```python
from build123d import *

# Parameters (mm, degrees)
BOSS_EXTRUDE2_DEPTH = 10
SKETCH2_W           = 6
SKETCH2_H           = 21.5
CUT_EXTRUDE1_DEPTH  = 2
SKETCH18_W          = 10
SKETCH18_H          = 4
CUT_EXTRUDE6_DEPTH  = 2.32
BOSS_EXTRUDE4_DEPTH = 35.965
SKETCH20_W          = 10
SKETCH20_H          = 4.318
BOSS_EXTRUDE5_DEPTH = 9
SKETCH21_W          = 2
SKETCH21_H          = 57.465
BOSS_EXTRUDE6_DEPTH = 0.889
BOSS_EXTRUDE7_DEPTH = 9.02
CUT_EXTRUDE7_DEPTH  = 1.016
SKETCH24_W          = 4.069
SKETCH24_H          = 2.54
CUT_EXTRUDE8_DEPTH  = 1
SKETCH30_R          = 0.75565
CUT_EXTRUDE14_DEPTH = 95.738007626
SKETCH34_R          = 1.5
CUT_EXTRUDE18_DEPTH = 10
SKETCH35_R          = 0.75
CUT_EXTRUDE19_DEPTH = 60.59814159
SKETCH36_W          = 6
SKETCH36_H          = 10
CUT_EXTRUDE20_DEPTH = 10
SKETCH37_W          = 9
SKETCH37_H          = 2
BOSS_EXTRUDE8_DEPTH = 3.65
SKETCH38_W          = 4.069
SKETCH38_H          = 10
BOSS_EXTRUDE9_DEPTH = 3
SKETCH39_R          = 0.75
CUT_EXTRUDE21_DEPTH = 3


with BuildPart() as part:
    # Sketch1 → Boss-Extrude2 (new body)
    with BuildSketch(Plane.XY):
        Polygon((-4, 0), (-0.82, 0), (-0.82, 21.5), (-6.32, 21.5), (-6.32, 17.5), (-4, 17.5), align=None)
    extrude(amount=BOSS_EXTRUDE2_DEPTH)

    # Sketch2 → Cut-Extrude1 (cut)
    with BuildSketch(Plane(origin=(-0.82, 0, 0), x_dir=(0, 0, -1), z_dir=(1, 0, 0))):
        with Locations((-5, 10.75)):
            Rectangle(SKETCH2_W, SKETCH2_H)
    extrude(amount=-CUT_EXTRUDE1_DEPTH, mode=Mode.SUBTRACT)

    # Sketch18 → Cut-Extrude6 (cut)
    with BuildSketch(Plane.ZY.offset(6.32)):
        with Locations((5, 19.5)):
            Rectangle(SKETCH18_W, SKETCH18_H)
    extrude(amount=-CUT_EXTRUDE6_DEPTH, mode=Mode.SUBTRACT)

    # Sketch19 → Boss-Extrude4 (add)
    with BuildSketch(Plane(origin=(0, 21.5, 0), x_dir=(1, 0, 0), z_dir=(0, 1, 0))):
        Polygon((-0.82, -10), (-4, -10), (-4, 0), (-0.82, 0), (-0.82, -2), (-2.82, -2), (-2.82, -8), (-0.82, -8), align=None)
    extrude(amount=BOSS_EXTRUDE4_DEPTH)

    # Sketch20 → Boss-Extrude5 (add)
    with BuildSketch(Plane.ZY.offset(4)):
        with Locations((5, 55.306)):
            Rectangle(SKETCH20_W, SKETCH20_H)
    extrude(amount=BOSS_EXTRUDE5_DEPTH)

    # Sketch21 → Boss-Extrude6 (add)
    with BuildSketch(Plane(origin=(-0.82, 0, 0), x_dir=(0, 0, -1), z_dir=(1, 0, 0))):
        with Locations((-9, 28.7325)):
            Rectangle(SKETCH21_W, SKETCH21_H)
        with Locations((-1, 28.7325)):
            Rectangle(SKETCH21_W, SKETCH21_H)
    extrude(amount=BOSS_EXTRUDE6_DEPTH)

    # Sketch22 → Boss-Extrude7 (add)
    with BuildSketch(Plane.XZ):
        Polygon((-4, 10), (0.069, 10), (0.069, 8), (-2.82, 8), (-2.82, 2), (0.069, 2), (0.069, 0), (-4, 0), align=None)
    extrude(amount=BOSS_EXTRUDE7_DEPTH)

    # Sketch23 → Cut-Extrude7 (cut)
    with BuildSketch(Plane.XY.offset(10)):
        Polygon((0.069, -3.02), (0.069, -4.29), (-4, -4.29), (-4, -1.75), (0.069, -1.75), align=None)
        Polygon((-4, 47.426731456), (-4, 48.696731456), (0.069, 48.696731456), (0.069, 46.156731456), (-4, 46.156731456), align=None)
    extrude(amount=-CUT_EXTRUDE7_DEPTH, mode=Mode.SUBTRACT)

    # Sketch24 → Cut-Extrude8 (cut)
    with BuildSketch(Plane.XY.offset(10)):
        with Locations((-1.9655, 35.355048592)):
            Rectangle(SKETCH24_W, SKETCH24_H)
    extrude(amount=-CUT_EXTRUDE8_DEPTH, mode=Mode.SUBTRACT)

    # Sketch30 → Cut-Extrude14 (cut, through all)
    with BuildSketch(Plane(origin=(35.063086629, -23.678267082, 9), x_dir=(1, 0, 0), z_dir=(0, 0, 1))):
        with Locations((-36.581586629, 59.033315674)):
            Circle(SKETCH30_R)
    extrude(amount=-CUT_EXTRUDE14_DEPTH, mode=Mode.SUBTRACT)

    # Sketch34 → Cut-Extrude18 (cut)
    with BuildSketch(Plane(origin=(0, 57.465, 0), x_dir=(1, 0, 0), z_dir=(0, 1, 0))):
        with Locations(Location((-9.5, -5, 0), (0, 0, 270))):
            Circle(SKETCH34_R)
    extrude(amount=-CUT_EXTRUDE18_DEPTH, mode=Mode.SUBTRACT)

    # Sketch35 → Cut-Extrude19 (cut, through all)
    with BuildSketch(Plane.XY.offset(8.984)):
        with Locations((-1.5185, 47.456731456)):
            Circle(SKETCH35_R)
        with Locations((-1.5185, -3.05)):
            Circle(SKETCH35_R)
    extrude(amount=-CUT_EXTRUDE19_DEPTH, mode=Mode.SUBTRACT)

    # Sketch36 → Cut-Extrude20 (cut)
    with BuildSketch(Plane(origin=(-2.82, 0, 0), x_dir=(0, 0, -1), z_dir=(1, 0, 0))):
        with Locations((-5, 48.147)):
            Rectangle(SKETCH36_W, SKETCH36_H)
    extrude(amount=-CUT_EXTRUDE20_DEPTH, mode=Mode.SUBTRACT)

    # Sketch37 → Boss-Extrude8 (add)
    with BuildSketch(Plane.XZ.offset(-53.147)):
        with Locations((-8.5, 9)):
            Rectangle(SKETCH37_W, SKETCH37_H)
        with Locations((-8.5, 1)):
            Rectangle(SKETCH37_W, SKETCH37_H)
    extrude(amount=BOSS_EXTRUDE8_DEPTH)

    # Sketch38 → Boss-Extrude9 (add)
    with BuildSketch(Plane.XZ.offset(9.02)):
        with Locations((-1.9655, 5)):
            Rectangle(SKETCH38_W, SKETCH38_H)
    extrude(amount=-BOSS_EXTRUDE9_DEPTH)

    # Sketch39 → Cut-Extrude21 (cut)
    with BuildSketch(Plane.XZ.offset(9.02)):
        with Locations(Location((-1.7, 5, 0), (0, 0, 270))):
            Circle(SKETCH39_R)
    extrude(amount=-CUT_EXTRUDE21_DEPTH, mode=Mode.SUBTRACT)


solid = part.part
```
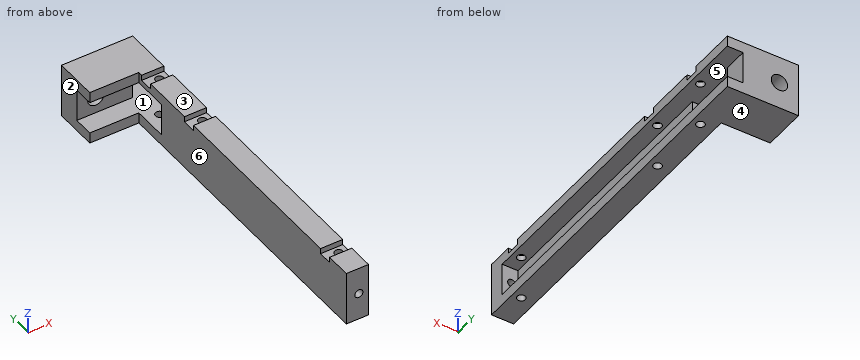
The listing builds one solid part. Answer for the finished solid, in the listing's coordinates (mm). Face numbers are marked on the shaded views. A direction names the side the tool comes from. Coordinates: 2 decimals unless noted, no trailing zeros. Loops run counter-clockwise (first coordinate to the right, second up) from the corner with the lowest first, then second, coordinate; pieces in that order, holes last. Notation, with made-up numbers: M 31.25,19.5 L 38.25,19.5 A22 cw 38.25,50.5 Z; hole C -39,43 d1. An arc over 180 degrees is marked long. Answer as a JSON object with one key per item and string values. Group by question number.
Item 1: Which of the six approach directions +Z, -Z, +X, -X, +Y, -Y give full straight-line access (tool end or side, diameter ignored) to the marked faces 4, 5 and 6?
Item 2: Section C-C (z = 5) is taken. Write down the section's boundary in (x, y) (3 decimals), and give its area (3 significant figures).
Item 3: Consider L1, parallel to Y at x = -1.5, z = 1.5 (1 decimal); L2, parallel to Y at x = -3.5, z = 5.5 (3 decimals); L3, parallel to X at y = -7.4, z = 5. Determine where each line is inside the solid, lowest interval first.
Item 4: Section B-B (y = -3.05) is taken. Write down the section's boundary in (x, z), and give its area (3 significant figures).
Item 5: Each of these flat-tipped pins is pushed along its axis until it touches: P1, Ø1.3, axis at y = 54.5, z = 5, coming from the +X side; P2, Ø1.3, axis at x = -2, y = 47.5, coming from the +Z side; P3, Ø2, axis at y = 34, z = 5, coming from the -X side. Where does it stop, or does it pass through?
Item 6: Section D-D (z = 1) is taken. Give the number of separate pieces and of enclosed holes in the cut face, and give its area (3 significant figures).
Item 7: Determine the mould class of the marked faces 1, 2 and 3 for opening direction Z: +Z half, -Z half, draft (parallel to the pull), parting line (faces both ways), or undercut.
Item 8: Section A-A (x = -9.5) is taken. Write down the section's boundary in (y, z) (3 decimals).
Solved:
{
 "1": {"face 4": "-Z, +X, -X, +Y, -Y", "face 5": "+X", "face 6": "+Z, -Z, -X, -Y"},
 "2": {"outline": "M -13,53.147 L -11,53.147 L -11,57.465 L -13,57.465 Z; M -8,53.147 L -2.82,53.147 L -2.82,57.465 L -8,57.465 Z; M -4,-9.02 L -2.45,-9.02 L -2.45,-6.02 L -2.82,-6.02 L -2.82,43.147 L -4,43.147 Z; M -0.95,-9.02 L 0.069,-9.02 L 0.069,-6.02 L -0.95,-6.02 Z", "area": "96.7 mm2"},
 "3": {"L1": "y = -9 to -3.8, -2.3 to 34.6, 36.1 to 46.7, 48.2 to 57.5", "L2": "y = -9.02 to 43.147, 53.147 to 57.465", "L3": "x = -4 to -2.45, -0.95 to 0.07"},
 "4": {"outline": "M -4,0 L -2.27,0 L -2.27,2 L -2.82,2 L -2.82,8 L -2.27,8 L -2.27,8.98 L -4,8.98 Z; M -0.77,0 L 0.07,0 L 0.07,2 L -0.77,2 Z; M -0.77,8 L 0.07,8 L 0.07,8.98 L -0.77,8.98 Z", "area": "14.7 mm2"},
 "5": {"P1": "stops at x = -2.82", "P2": "stops at z = 8.98", "P3": "stops at x = -4"},
 "6": {"separate pieces": "1", "enclosed holes": "3", "area": "337 mm2"},
 "7": {"face 1": "undercut", "face 2": "draft", "face 3": "+Z half"},
 "8": {"outline": "M 49.497,0 L 57.465,0 L 57.465,3.5 L 53.147,3.5 L 53.147,2 L 49.497,2 Z; M 49.497,8 L 53.147,8 L 53.147,6.5 L 57.465,6.5 L 57.465,10 L 49.497,10 Z"}
}
